Part print with two shaded views. Sizes in mm from the minimum x, y, z corner. A direction names the side the tool comes from. Round coordinates to 2 decimals unless told otherwise and drop trailing zeros. Write each loop counter-clockwise with the first axis right and the second up, starting at its lowest first coordinate (ties: lowest second). Pieces come first, ordered by that corner, then holes. Notation, with made-up numbers: (-13, 57.5) -> (7, 57.5) arc R27 ccw to (7, 77.5) -> close; hole circle Ø7 at (-12, 2.5). An arc over 180 degrees is marked (long way). Return JSON: item names as keys, results as strings. Group by question number.
(1) Mould opens along Y. For the marked faces 3, 4, 5 and 6 say: +Y half, -Y half, draft (parallel to the pull), parting line (faces both ways), or undercut.
(2) Saw through at C-C (y = 28). List the corners of the cut face in (x, z).
(3) Drop flat-ended pins along their axis: pin 1 Ø6 at (y, z) = (70, 116.5) entering from +X; pin 2 Ø23 at (x, z) = (31.75, 95.25) entering from +Y; pin 3 Ø6 at (y, z) = (68, 73.5) entering from +X; pin 4 Ø8 at (x, y) = (17, 99.5) entering from -Z. Give the stop position or say it passes through.
(4) Saw through at A-A (z = 31.75). List the corners of the cut face in (x, y), plus the area to 3 significant figures.
(5) Tool access for the marked faces 1 and 2: list every direction of +Z, -Z, +X, -X, +Y, -Y with a clear straight run to the whole face (end or side of a thin tool).
(6) Saw through at D-D (z = 68). List the corners of the cut face in (x, y), plus the area to 3 significant figures.
(7) Saw through at B-B (x = 31.75). List the corners of the cut face in (y, z).
(8) Drill centre lines: L1, parallel to X at y = 51, z = 31; L2, parallel to Z at x = 95, y = 61; L3, parallel to Z at x = 31.75, y = 30.5. Where is each one in solid material? Low to high. Write a range as from..to.
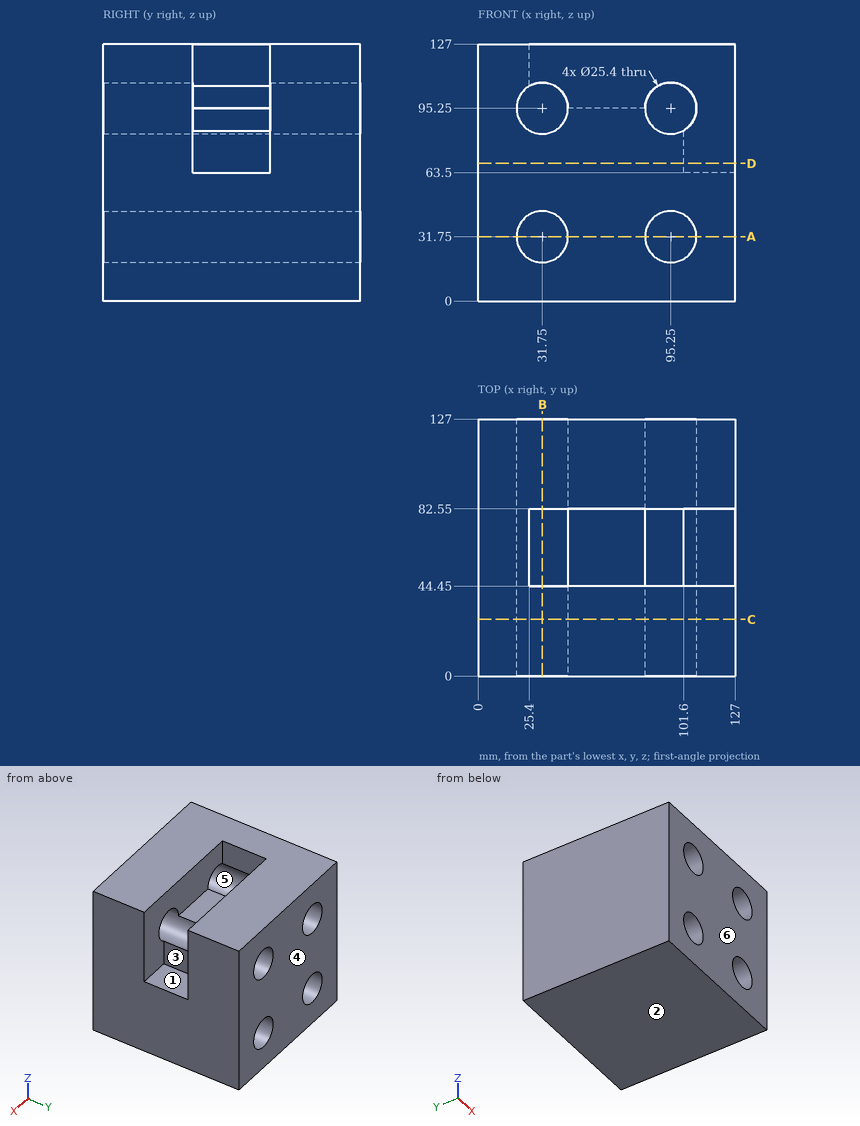
Computed values:
{
 "1": {"face 3": "undercut", "face 4": "+Y half", "face 5": "draft", "face 6": "-Y half"},
 "2": {"outline": "(0, 0) -> (127, 0) -> (127, 127) -> (0, 127) -> close; hole circle Ø25.4 at (31.75, 31.75); hole circle Ø25.4 at (31.75, 95.25); hole circle Ø25.4 at (95.25, 31.75); hole circle Ø25.4 at (95.25, 95.25)"},
 "3": {"pin 1": "x = 25.4", "pin 2": "through", "pin 3": "x = 101.6", "pin 4": "z = 0"},
 "4": {"outline": "(0, 0) -> (19.05, 0) -> (19.05, 127) -> (0, 127) -> close; (44.45, 0) -> (82.55, 0) -> (82.55, 127) -> (44.45, 127) -> close; (107.95, 0) -> (127, 0) -> (127, 127) -> (107.95, 127) -> close", "area": "9,680 mm2"},
 "5": {"face 1": "+Z, +X", "face 2": "-Z, +X, -X, +Y, -Y"},
 "6": {"outline": "(0, 0) -> (127, 0) -> (127, 44.45) -> (101.6, 44.45) -> (101.6, 82.55) -> (127, 82.55) -> (127, 127) -> (0, 127) -> close", "area": "15,200 mm2"},
 "7": {"outline": "(0, 0) -> (127, 0) -> (127, 19.05) -> (0, 19.05) -> close; (0, 44.45) -> (127, 44.45) -> (127, 82.55) -> (0, 82.55) -> close; (0, 107.95) -> (44.45, 107.95) -> (44.45, 127) -> (0, 127) -> close; (82.55, 107.95) -> (127, 107.95) -> (127, 127) -> (82.55, 127) -> close"},
 "8": {"L1": "0..19.07, 44.43..82.57, 107.93..127", "L2": "0..19.05, 44.45..82.55", "L3": "0..19.05, 44.45..82.55, 107.95..127"}
}
